Here's how the part is built. I have some questions about the finished solid (model axes, mm). Face numbers are marked on the shaded views. A direction names the side the tool comes from. Give positions to 0.01 mm unless a question says otherwise; leave off trailing zeros. Write each loop counter-clockwise with the first axis right and the second up, starting at its lowest first coordinate (ties: lowest second). Pieces come first, ordered by that corner, then holes. Notation, with made-up numbers: (-18.5, 87) - (11.5, 87) arc R20 ccw to (11.5, 122) - close; hole circle Ø3 at (75, -23). An arc over 180 degrees is marked (long way). Use a Markdown table: item, result.
```python
from build123d import *

# Parameters (mm, degrees)
F0_R     = 0.381
F1_DEPTH = 0.7366
F2_DEPTH = 3.556
F3_SCALE = 7.5


with BuildPart() as f1:
    # F0 (on Front) → F1 (new body)
    with BuildSketch(Plane.XZ):
        Polygon((-3.4709807732, 23.1845746487), (-6.6709807732, 23.1845746487), (-6.6709807732, 16.1845746487), (0.1870192268, 16.1845746487), (0.1870192268, 18.9785746487), (-1.704775727, 20.2454317916), align=None)
        with Locations((-5.3821913898, 17.5259150565)):
            Circle(F0_R, mode=Mode.SUBTRACT)
        with Locations((-5.4190722294, 20.4617753625)):
            Circle(F0_R, mode=Mode.SUBTRACT)
    extrude(amount=F1_DEPTH)

    # F0 (on Front) → F2 (join)
    with BuildSketch(Plane.XZ):
        with Locations((-5.4190722294, 20.4617753625)):
            Circle(F0_R)
    extrude(amount=F2_DEPTH)


with BuildPart() as f1_1:
    # F3: moved
    add(f1.part.scale(F3_SCALE))


solid = f1_1.part
```
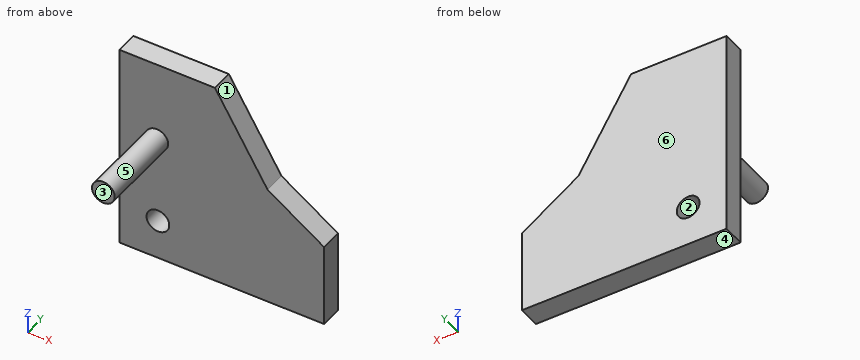
Item 1: Thinking about a two-plate mould opening in Z: for the marked faces 1, 2, 3 and 4, which applies, +Z half, -Z half, draft (parallel to the pull), parting line (faces both ways), or undercut?
Values:
| item | result |
|---|---|
| face 1 | +Z half |
| face 2 | undercut |
| face 3 | draft |
| face 4 | -Z half |
Item 2: I need wall thicknesses on line 1 along Y through (x, z) = (-16, 147.5); line 2 along Z through (x, y) = (-41, -2.5); line 3 along X through (y, z) = (-6.5, 152). Which ranges of each line are inside material? Lowest first, please. Write a range as [from, to].
Values:
| item | result |
|---|---|
| line 1 | y = [-5.52, 0] |
| line 2 | z = [121.38, 128.66], [134.23, 173.88] |
| line 3 | x = [-43.1, -38.19] |
Item 3: If we section it at B-B, the plane x = -29: Write out the boundary of the cut face in (y, z).
Values:
| item | result |
|---|---|
| outline | (-5.52, 121.38) - (0, 121.38) - (0, 173.88) - (-5.52, 173.88) - close |
Item 4: If we section it at A-A, the plane z = 133: Write out the boundary of the cut face in (x, y), plus the area to 3 significant figures.
Values:
| item | result |
|---|---|
| outline | (-50.03, -5.52) - (-42.76, -5.52) - (-42.76, 0) - (-50.03, 0) - close; (-37.97, -5.52) - (1.4, -5.52) - (1.4, 0) - (-37.97, 0) - close |
| area | 258 mm2 |
Item 5: Will these pins go through, and if not, where does the flat tip stop? pin 1 Ø1 at (y, z) = (-24, 149) entering from +X; pin 2 Ø15.5 at (x, z) = (-12, 144) entering from -Y.
Values:
| item | result |
|---|---|
| pin 1 | passes through |
| pin 2 | stops at y = -5.52 |
Item 6: If we section it at C-C, the plane z = 152.5: Write out the boundary of the cut face in (x, y), plus the area to 3 significant figures.
Values:
| item | result |
|---|---|
| outline | (-50.03, -5.52) - (-43.33, -5.52) - (-43.33, -26.67) - (-37.95, -26.67) - (-37.95, -5.52) - (-13.18, -5.52) - (-13.18, 0) - (-50.03, 0) - close |
| area | 317 mm2 |
Item 7: If we section it at D-D, the plane y = -18.75: Write out the boundary of the cut face in (x, z) (1 decimal).
Values:
| item | result |
|---|---|
| outline | circle Ø5.7 at (-40.6, 153.5) |
Item 8: For the marked faces 5 and 6, which set-ups out of +Z, -Z, +X, -X, +Y, -Y let a thin tool reach every point of the face, with its end or its side?
Values:
| item | result |
|---|---|
| face 5 | -Y |
| face 6 | +Z, -Z, +X, -X, +Y |
